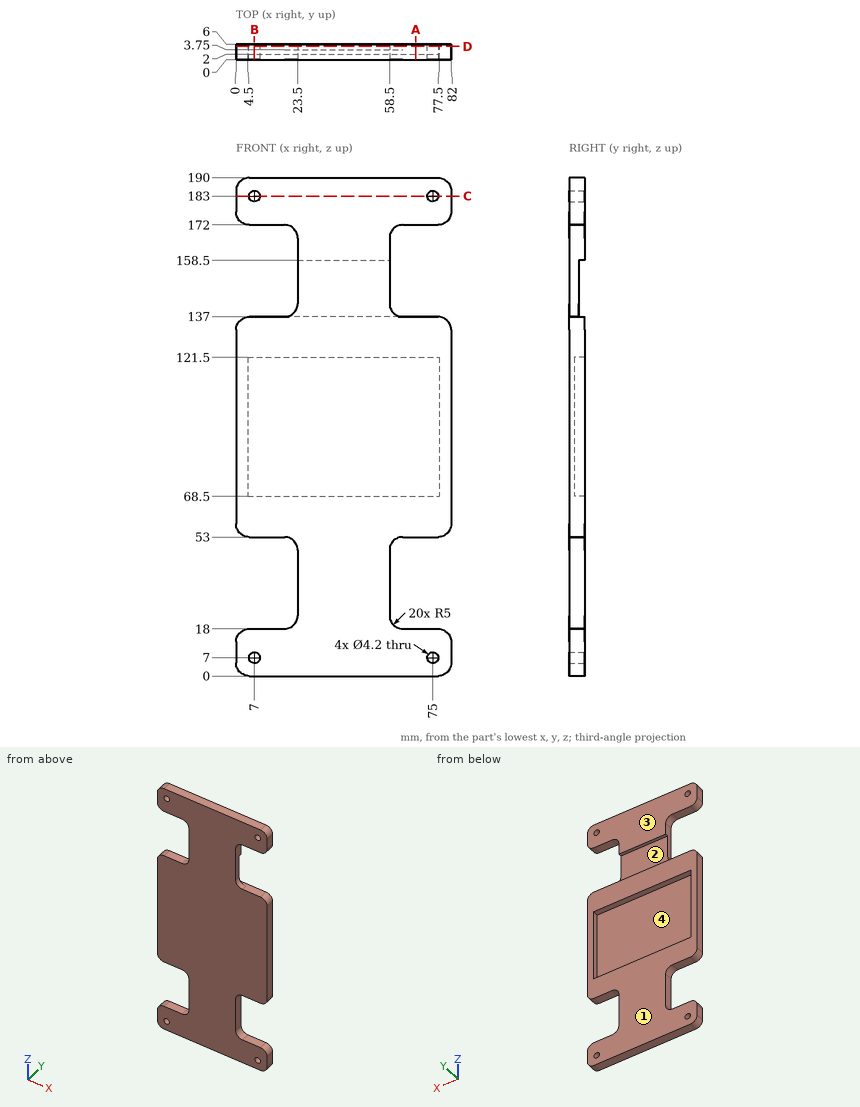
Answer from the drawing. Dimensions are ordinates in mm from the lowest x, y and z of the part. A direction names the side the tool comes from. Coordinates: 2 decimals unless noted, no trailing zeros. Write each loop counter-clockwise with the first axis right and the second up, starting at its lowest first coordinate (ties: lowest second). Pieces come first, ordered by that corner, then holes. Notation, with made-up numbers: (0, 63.25) - (15, 63.25) arc R22 ccw to (15, 81.25) - close; hole circle Ø10 at (33.5, 48.25). An arc over 180 degrees is marked (long way). One line per question, with ' | ' between items.
Q1. Find section A-A, the plane x = 68.5. Write down the section's boundary in (y, z), plus the area to 3 significant figures.
Result set:
outline: (0, 0) - (6, 0) - (6, 18) - (0, 18) - close; (0, 53) - (6, 53) - (6, 68.5) - (2, 68.5) - (2, 121.5) - (6, 121.5) - (6, 137) - (0, 137) - close; (0, 172) - (6, 172) - (6, 190) - (0, 190) - close | area: 508 mm^2
Q2. For the marked faces 1 and 2, determine the directions among +Z, -Z, +X, -X, +Y, -Y from which every point of the face is accessible in a straight line to the end or side of a thin tool.
Result set:
face 1: +Z, -Z, +X, -X, +Y | face 2: +X, -X, +Y
Q3. Determine the mould class of the marked faces 3 and 4 for opening direction Z: +Z half, -Z half, draft (parallel to the pull), parting line (faces both ways), or undercut.
Result set:
face 3: draft | face 4: undercut
Q4. Find section B-B, the plane x = 7. Write down the section's boundary in (y, z).
Result set:
outline: (0, 0) - (6, 0) - (6, 4.9) - (0, 4.9) - close; (0, 9.1) - (6, 9.1) - (6, 18) - (0, 18) - close; (0, 53) - (6, 53) - (6, 68.5) - (2, 68.5) - (2, 121.5) - (6, 121.5) - (6, 137) - (0, 137) - close; (0, 172) - (6, 172) - (6, 180.9) - (0, 180.9) - close; (0, 185.1) - (6, 185.1) - (6, 190) - (0, 190) - close
Q5. Each of these flat-tipped pins is pushed along its axis until it touches: P1, Ø12, axis at x = 22, z = 103.5, coming from the +Y side; P2, Ø17, axis at x = 33, z = 149, coming from the +Y side; P3, Ø6, axis at x = 44.5, z = 108, coming from the -Y side; P4, Ø2.5, axis at x = 75, z = 183, coming from the -Y side. Where does it stop, or does it pass through?
Result set:
P1: y = 2 | P2: y = 3.75 | P3: y = 0 | P4: through
Q6. Find section D-D, the plane y = 5.05. State how many separate pieces and enclosed holes the cut face has, plus the area to 3 significant figures.
Result set:
separate pieces: 2 | enclosed holes: 5 | area: 7,580 mm^2
Q7. Consider L1, parallel to Z at x = 75, y = 2.55; L2, parallel to X at y = 1.3, z = 183; L3, parallel to Z at x = 7, y = 1.45. Determine where each line is inside the solid, lowest interval first. Write a range as [from, to].
Result set:
L1: [0, 4.9], [9.1, 18], [53, 68.5], [121.5, 137], [172, 180.9], [185.1, 190] | L2: [0, 4.9], [9.1, 72.9], [77.1, 82] | L3: [0, 4.9], [9.1, 18], [53, 137], [172, 180.9], [185.1, 190]
Q8. Find section C-C, the plane z = 183. Write down the section's boundary in (x, y), plus the area to 3 significant figures.
Result set:
outline: (0, 0) - (4.9, 0) - (4.9, 6) - (0, 6) - close; (9.1, 0) - (72.9, 0) - (72.9, 6) - (9.1, 6) - close; (77.1, 0) - (82, 0) - (82, 6) - (77.1, 6) - close | area: 442 mm^2
